```python
from build123d import *

# Parameters (mm, degrees)
SKETCH_1_R               = 50
EXTRUDE_1_DEPTH          = 50
CUT_EXTRUDE_1_DEPTH      = 15
CUT_EXTRUDE_1_DEPTH_BACK = 15
SKETCH_2_OUTSIDE_W       = 132
SKETCH_2_OUTSIDE_H       = 132
SKETCH_2_OUTSIDE_R       = 40
CUT_EXTRUDE_2_DEPTH      = 76
CUT_EXTRUDE_2_DEPTH_BACK = 76
SKETCH_3_R               = 10


with BuildPart() as part:
    # 草图1 → 凸台-拉伸1 (new body)
    with BuildSketch(Plane.XY):
        Circle(SKETCH_1_R)
    extrude(amount=EXTRUDE_1_DEPTH)

    # 草图2 outside → 切除-拉伸1 (cut, two sides: drawn at the far end of the back side and taken through both)
    with BuildSketch(Plane.XY.offset(25).offset(-CUT_EXTRUDE_1_DEPTH_BACK)):
        Rectangle(SKETCH_2_OUTSIDE_W, SKETCH_2_OUTSIDE_H)
        Circle(SKETCH_2_OUTSIDE_R, mode=Mode.SUBTRACT)
    extrude(amount=CUT_EXTRUDE_1_DEPTH + CUT_EXTRUDE_1_DEPTH_BACK, mode=Mode.SUBTRACT)

    # 草图3 → 切除-拉伸2 (cut, two sides: drawn at the far end of the back side and taken through both)
    with BuildSketch(Plane.XY.offset(25).offset(-CUT_EXTRUDE_2_DEPTH_BACK)):
        Circle(SKETCH_3_R)
    extrude(amount=CUT_EXTRUDE_2_DEPTH + CUT_EXTRUDE_2_DEPTH_BACK, mode=Mode.SUBTRACT)


solid = part.part
```
Geometry check sheet. Reference: the model listing, model coordinates, mm. A direction names the side the tool comes from. Coordinates: 2 decimals unless noted, no trailing zeros. Loops run counter-clockwise (first coordinate to the right, second up) from the corner with the lowest first, then second, coordinate; pieces in that order, holes last. Notation, with made-up numbers: (6, 2.5) - (21, 2.5) arc R20 cw to (21, 27.5) - close; hole circle Ø1 at (70, 25). An arc over 180 degrees is marked (long way). One line per item, written item: value. Start each with the question number.
(1) Cross-section at C-C on z = 38. Enter the section's corners in (x, y).
(2) Mould release check, pull along Z, two halves, no side actions. Record for faces 3 (the cylindrical face through (-8.67, -39.05, 24.79)), 4 (the flat face through (-0.7, -10.4, 50)), 5 (the cylindrical face through (47.69, 15.02, 44.93)): released by +Z, released by -Z, zero draft, split by the parting line, or undercut.
(3) Tool access check on faces 1 (the flat face through (-22, 34, 10)), 2 (the cylindrical face through (-2.17, -9.76, 24.65)). Record the directions out of +Z, -Z, +X, -X, +Y, -Y that give a thin tool (end or side, any length) a straight path to the whole face; none if there is none.
(4) Cross-section at D-D on x = -37.5. Enter the section's corners in (y, z).
(5) Depth check by flat-ended pin: P1, Ø4, axis at y = 16, z = 16, coming from the +X side; P2, Ø4, axis at x = 4, z = 5, coming from the -Y side; P3, Ø3, axis at x = 21, z = 29.5, coming from the -Y side; P4, Ø18, axis at x = 0, y = 0, coming from the +Z side. Enter the tip coordinate at first touch or a pass-through.
(6) Material ranges on line 1 (Z direction, x = -30, y = -35.5); line 2 (Y direction, x = 0, z = 16); line 3 (Y direction, x = 2, z = 23), recorded low to high. Write a range as [from, to].
(7) Cross-section at A-A on y = 0. Enter the section's corners in (x, z), plus the area to 3 significant figures.
Results below:
1. outline: circle Ø80 at (0, 0); hole circle Ø20 at (0, 0)
2. face 3: undercut
2. face 4: released by +Z
2. face 5: zero draft
3. face 1: none
3. face 2: +Z, -Z
4. outline: (-33.07, 0) - (33.07, 0) - (33.07, 10) - (13.92, 10) - (13.92, 40) - (33.07, 40) - (33.07, 50) - (-33.07, 50) - (-33.07, 40) - (-13.92, 40) - (-13.92, 10) - (-33.07, 10) - close
5. P1: stops at x = 37.47
5. P2: stops at y = -49.96
5. P3: stops at y = -34.92
5. P4: passes through
6. line 1: z = [0, 10], [40, 50]
6. line 2: y = [-40, -10], [10, 40]
6. line 3: y = [-39.95, -9.8], [9.8, 39.95]
7. outline: (-50, 0) - (-10, 0) - (-10, 50) - (-50, 50) - (-50, 40) - (-40, 40) - (-40, 10) - (-50, 10) - close; (10, 0) - (50, 0) - (50, 10) - (40, 10) - (40, 40) - (50, 40) - (50, 50) - (10, 50) - close
7. area: 3,400 mm2
